```python
from build123d import *

# Parameters (mm, degrees)
F0_W     = 909
F0_H     = 81
F1_DEPTH = 549
F2_W     = 909
F2_H     = 176
F3_DEPTH = 25
F4_W     = 1100
F4_H     = 450
F5_DEPTH = 300


with BuildPart() as f1:
    # F0 (on Top) → F1 (new body)
    with BuildSketch(Plane.XY):
        Rectangle(F0_W, F0_H)
    extrude(amount=F1_DEPTH)

    # F2 (on face) → F3 (join)
    with BuildSketch(Plane(origin=(0, 0, 0), x_dir=(1, 0, 0), z_dir=(0, 0, -1))):
        Rectangle(F2_W, F2_H)
    extrude(amount=-F3_DEPTH)

    # F4 (on face) → F5 (join)
    with BuildSketch(Plane(origin=(0, 0, 0), x_dir=(1, 0, 0), z_dir=(0, 0, -1))):
        Rectangle(F4_W, F4_H)
    extrude(amount=F5_DEPTH)


solid = f1.part
```
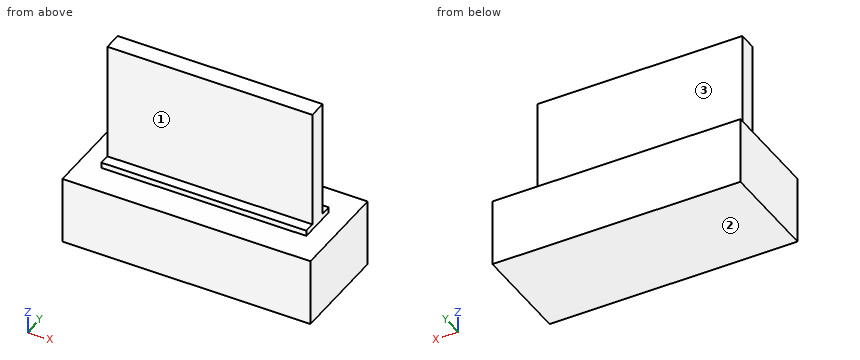
Geometry check sheet. Reference: the model listing, model coordinates, mm. Face numbers are marked on the shaded views. A direction names the side the tool comes from. Round coordinates to 2 decimals unless told otherwise and drop trailing zeros. Loops run counter-clockwise (first coordinate to the right, second up) from the corner with the lowest first, then second, coordinate; pieces in that order, holes last. Notation, with made-up numbers: (-3.5, -22.75) - (9.5, -22.75) arc R26 ccw to (9.5, 8.25) - close; hole circle Ø9 at (-12, 45.5). An arc over 180 degrees is marked (long way). Write each question's results on one line, items separated by ' | '. Start each with the question number.
Q1. Cross-section at D-D on y = 158.5. Enter the section's corners in (x, z).
Q2. Cross-section at B-B on x = 131.5. Enter the section's corners in (y, z).
Q3. Cross-section at C-C on z = 365. Enter the section's corners in (x, y), and give its area (3 significant figures).
Q4. Cross-section at A-A on y = -60. Enter the section's corners in (x, z), and give its area (3 significant figures).
Q5. Thickness scan on line 1 (X direction, y = 30, z = 405.5); line 2 (Z direction, x = -461, y = -58); line 3 (Z direction, x = 310, y = -69). Record the ranges inside material, lowest first. Write a range as [from, to].
Q6. Access from +Z, -Z, +X, -X, +Y, -Y to the whole of each face (thin tool, end or side, straight path). Record for the marked faces 1, 2 and 3.
Q7. Gauge pin test, flat ends, axial feed: P1, Ø12.5, axis at x = -206.5, z = 13, coming from the -Y side; P2, Ø12.5, axis at x = 108.5, z = 10, coming from the +Y side; P3, Ø10, axis at x = -51.5, z = 407, coming from the +Y side. Record the tip position at first contact, or that the pin passes through.
Answers below:
1) outline: (-550, -300) - (550, -300) - (550, 0) - (-550, 0) - close
2) outline: (-225, -300) - (225, -300) - (225, 0) - (88, 0) - (88, 25) - (40.5, 25) - (40.5, 549) - (-40.5, 549) - (-40.5, 25) - (-88, 25) - (-88, 0) - (-225, 0) - close
3) outline: (-454.5, -40.5) - (454.5, -40.5) - (454.5, 40.5) - (-454.5, 40.5) - close | area: 73,600 mm²
4) outline: (-550, -300) - (550, -300) - (550, 0) - (454.5, 0) - (454.5, 25) - (-454.5, 25) - (-454.5, 0) - (-550, 0) - close | area: 353,000 mm²
5) line 1: x = [-454.5, 454.5] | line 2: z = [-300, 0] | line 3: z = [-300, 25]
6) face 1: +Z, +X, -X, -Y | face 2: -Z, +X, -X, +Y, -Y | face 3: +Z, +X, -X, +Y
7) P1: stops at y = -88 | P2: stops at y = 88 | P3: stops at y = 40.5
